Can you work these out from the model? Positions are in its coordinate system, mm. Face numbers are marked on the shaded views. A direction names the side the tool comes from. Coordinates: 2 decimals unless noted, no trailing zeros. Order: outer loops, then holes, each group sorted by start corner. A loop starts at its lowest first (then second) coordinate and runs counter-clockwise, first axis right, second up. Notation, with made-up numbers: (79, 61) -> (114, 61) arc R9 ccw to (114, 69) -> close; hole circle Ø7 at (76.25, 3.5). An arc over 180 degrees is marked (long way). Return JSON: item names as keys, results as strings. Group by question number.
1) For the marked faces 1, 2 and 3, which set-ups out of +Z, -Z, +X, -X, +Y, -Y let a thin tool reach every point of the face, with its end or its side?
2) If we section it at D-D, the plane x = 5.75: Please give me the cut outline in (y, z), then the cut area to 3 significant figures.
3) If we section it at C-C, the plane y = 3.75: Please give me the cut outline in (x, z).
4) If we section it at A-A, the plane x = 15.75: Please give me the cut outline in (y, z), then the cut area to 3 significant figures.
5) Thinking about a two-plate mould opening in Y: for the marked faces 4, 5, 6 and 7, which applies, +Y half, -Y half, draft (parallel to the pull), parting line (faces both ways), or undercut?
6) If I drill on probe 1 along X at (y, z) = (5.5, 0.7); probe 2 along Y at (x, z) = (18.25, 1.1); probe 3 along X at (y, z) = (-1.75, 0.45), over which ranges is the centre line in solid material (lowest first)? Write a range as from..to.
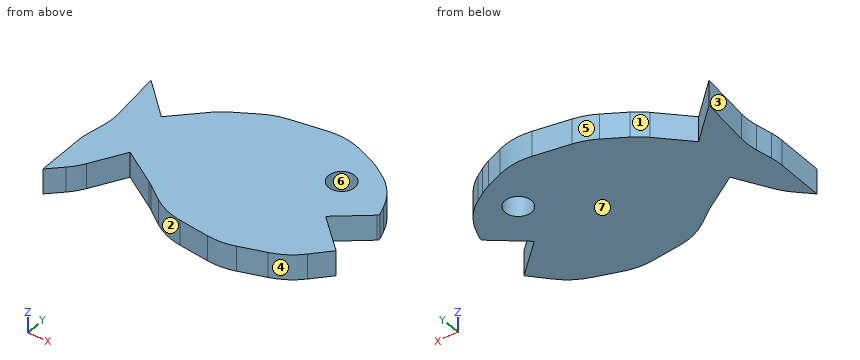
from build123d import *

# Parameters (mm, degrees)
F0_R     = 1.044961
F1_DEPTH = 2


with BuildPart() as f1:
    # F0 (on Top) → F1 (new body)
    with BuildSketch(Plane.XY):
        with BuildLine():
            Line((5.007722, 6.82725), (2.795858, 4.615385))
            Line((2.795858, 4.615385), (0, 7.278107))
            Line((0, 7.278107), (0.423993, 3.249794))
            ThreePointArc((0.423993, 3.249794), (0.445773, 2.488009), (0.351528, 1.731763))
            Line((0.351528, 1.731763), (0.099933, 0.492308))
            ThreePointArc((0.099933, 0.492308), (0.025046, -0.002516), (0, -0.502348))
            Line((0, -0.502348), (0, -4.231373))
            Line((0, -4.231373), (1.057963, -3.201267))
            ThreePointArc((1.057963, -3.201267), (1.511144, -2.695677), (1.89165, -2.133352))
            Line((1.89165, -2.133352), (3.402669, 0.463712))
            Line((3.402669, 0.463712), (6.210531, -1.298084))
            ThreePointArc((6.210531, -1.298084), (6.357115, -1.393674), (6.500264, -1.494334))
            Line((6.500264, -1.494334), (7.757519, -2.411716))
            ThreePointArc((7.757519, -2.411716), (8.894254, -3.033361), (10.15255, -3.342065))
            Line((10.15255, -3.342065), (12.532795, -3.606537))
            ThreePointArc((12.532795, -3.606537), (13.611706, -3.609293), (14.666091, -3.380534))
            Line((14.666091, -3.380534), (16.664257, -2.714479))
            ThreePointArc((16.664257, -2.714479), (17.796263, -2.170925), (18.757136, -1.362462))
            Line((18.757136, -1.362462), (20.014793, 0))
            Line((20.014793, 0), (17.352073, 2.485207))
            Line((17.352073, 2.485207), (19.902285, 4.525379))
            ThreePointArc((19.902285, 4.525379), (19.970428, 4.627975), (19.966333, 4.751071))
            Line((19.966333, 4.751071), (19.69989, 5.497113))
            ThreePointArc((19.69989, 5.497113), (18.906432, 6.925225), (17.694968, 8.021325))
            Line((17.694968, 8.021325), (17.023118, 8.453229))
            ThreePointArc((17.023118, 8.453229), (16.632537, 8.680065), (16.223079, 8.870728))
            Line((16.223079, 8.870728), (14.957098, 9.392014))
            ThreePointArc((14.957098, 9.392014), (13.601922, 9.738439), (12.203814, 9.695924))
            Line((12.203814, 9.695924), (9.375468, 9.208279))
            ThreePointArc((9.375468, 9.208279), (8.504739, 8.97573), (7.689901, 8.590649))
            Line((7.689901, 8.590649), (6.008156, 7.601387))
            ThreePointArc((6.008156, 7.601387), (5.483359, 7.246084), (5.007722, 6.82725))
        make_face()
        with Locations((16.005702, 6.011697)):
            Circle(F0_R, mode=Mode.SUBTRACT)
    extrude(amount=F1_DEPTH)


solid = f1.part
Result sheet:
{
 "1": {"face 1": "+Z, -Z, +Y", "face 2": "+Z, -Z, -Y", "face 3": "+Z, -Z, -X"},
 "2": {"outline": "(-1.01, 0) -> (7.44, 0) -> (7.44, 2) -> (-1.01, 2) -> close", "area": "16.9 mm2"},
 "3": {"outline": "(0.37, 0) -> (18.93, 0) -> (18.93, 2) -> (0.37, 2) -> close"},
 "4": {"outline": "(-3.02, 0) -> (5, 0) -> (5, 2) -> (-3.02, 2) -> close; (7.02, 0) -> (9.07, 0) -> (9.07, 2) -> (7.02, 2) -> close", "area": "20.1 mm2"},
 "5": {"face 4": "-Y half", "face 5": "+Y half", "face 6": "undercut", "face 7": "draft"},
 "6": {"probe 1": "x = 0.19..1.87, 3.68..15.09, 16.92..19.7", "probe 2": "y = -1.84..1.65, 3.2..7.61", "probe 3": "x = 0..2.11, 6.85..18.36"}
}
